Geometry: see drawing. Coordinates: mm, zero at the bounding-box minimum. A direction names the side the tool comes from. Coordinates: 2 decimals unless noted, no trailing zeros. Loops run counter-clockwise (first coordinate to the right, second up) from the corner with the lowest first, then second, coordinate; pieces in that order, holes last. Notation, with made-up numbers: (-31, 13) -> (-3, 13) arc R26 cw to (-3, 43) -> close; hole circle Ø9 at (14.5, 81.5). An arc over 180 degrees is marked (long way). Put each result on its own line as item: value. Start each with the question number.
1) Contact query for flat-ended pins moving along their axis: P1, Ø2, axis at x = 11.5, z = 1.5, coming from the -Y side; P2, Ø1, axis at y = 5, z = 5, coming from the +X side; P3, Ø3, axis at x = 83.5, y = 2, coming from the +Z side. Output: stop coordinate, or through.
2) Cut plane C-C (x = 10.5). Return the cut outline in (y, z), plus the area to 3 significant figures.
3) Cut plane A-A (y = 3). Return the cut outline in (x, z).
4) Set-up query: the marked faces 1, 2 and 3. Return all of +Z, -Z, +X, -X, +Y, -Y with unobstructed straight access to the full face (end or side cutting, diameter ignored); none if empty.
5) Material intervals for L1, parallel to Z at x = 78.5, y = 3.1; L2, parallel to Y at x = 90, z = 3.05; L3, parallel to X at y = 2.75, z = 0.4, sorted ascending.
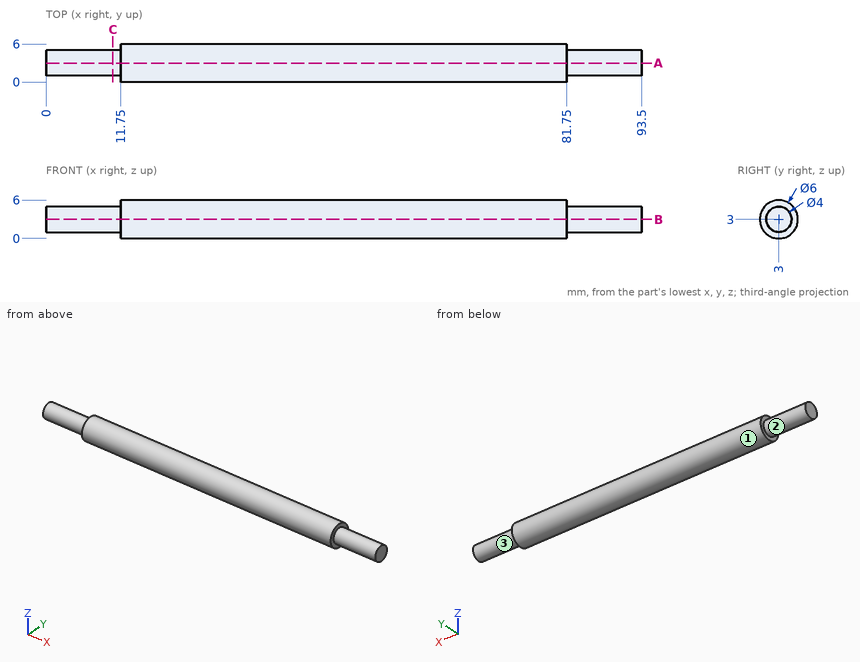
Results found:
1. P1: stops at y = 0.05
1. P2: stops at x = 81.75
1. P3: stops at z = 5
2. outline: circle Ø4 at (3, 3)
2. area: 12.6 mm2
3. outline: (0, 1) -> (11.75, 1) -> (11.75, 0) -> (81.75, 0) -> (81.75, 1) -> (93.5, 1) -> (93.5, 5) -> (81.75, 5) -> (81.75, 6) -> (11.75, 6) -> (11.75, 5) -> (0, 5) -> close
4. face 1: +X, -X
4. face 2: -X
4. face 3: +X
5. L1: z = 0 to 6
5. L2: y = 1 to 5
5. L3: x = 11.75 to 81.75
